Part model, mm, in its own coordinate system. A direction names the side the tool comes from. Give positions to 0.01 mm unless a question says otherwise; leave off trailing zeros. Order: outer loops, then holes, each group sorted by start corner. A loop starts at its lowest first (then second) coordinate and runs counter-clockwise, first axis right, second up. Notation, with made-up numbers: (66.5, 58) - (104.5, 58) arc R26 ccw to (104.5, 84) - close; hole circle Ø2 at (78, 85.5). An arc over 180 degrees is marked (long way). One line per item, written item: value.
```python
from build123d import *

# Parameters (mm, degrees)
BOSS_EXTRUDE1_DEPTH = 3


with BuildPart() as part:
    # Sketch1 → Boss-Extrude1 (new body)
    with BuildSketch(Plane.XY):
        Polygon((-112.34268018, 49.584121622), (-112.34268018, 23.584121622), (-115.34268018, 23.584121622), (-115.34268018, -26.415878378), (-112.34268018, -26.415878378), (-112.34268018, -52.415878378), (112.65731982, -52.415878378), (112.65731982, -26.415878378), (115.65731982, -26.415878378), (115.65731982, 23.584121622), (112.65731982, 23.584121622), (112.65731982, 49.584121622), align=None)
        with BuildLine():
            Line((13.274286272, -45.008836488), (13.301852176, -45.03203797))
            add(Edge.make_bspline(
                [(13.301852176, -45.03203797), (13.302434824, -45.031895887), (13.303594926, -45.031612989), (13.310345597, -45.026788399), (13.327424294, -45.013559601), (13.368373413, -44.979806794), (13.432345907, -44.924692433), (13.489247142, -44.874546261), (13.518732521, -44.84808225), (13.533463875, -44.834860418)],
                knots=[0, 0, 0, 0, 0.083775212, 0.166803477, 0.250583378, 0.499711324, 0.748903893, 0.874548479, 1, 1, 1, 1], degree=3))
            ThreePointArc((13.533463875, -44.834860418), (14.561847159, -43.83964014), (15.516962395, -42.773905432))
            ThreePointArc((15.516962395, -42.773905432), (30.145326147, -17.328936846), (35.253292189, 11.573383741))
            ThreePointArc((35.253292189, 11.573383741), (34.303607008, 26.14987852), (31.427393187, 40.471313366))
            ThreePointArc((31.427393187, 40.471313366), (30.556136604, 41.977838946), (29.052246095, 42.853636122))
            ThreePointArc((29.052246095, 42.853636122), (0.16598909, 46.766690687), (-28.731940535, 42.940791684))
            ThreePointArc((-28.731940535, 42.940791684), (-30.238466115, 42.069535101), (-31.114263292, 40.565644593))
            ThreePointArc((-31.114263292, 40.565644593), (-34.033665807, 26.252951242), (-35.027317855, 11.679387588))
            ThreePointArc((-35.027317855, 11.679387588), (-30.00656127, -17.238210094), (-15.455020905, -42.727190564))
            ThreePointArc((-15.455020905, -42.727190564), (-14.50312489, -43.795801606), (-13.477748449, -44.794119559))
            add(Edge.make_bspline(
                [(-13.477748449, -44.794119559), (-13.467950877, -44.802979196), (-13.448447729, -44.820615282), (-13.419486181, -44.846490582), (-13.372927905, -44.887713721), (-13.313203528, -44.93946889), (-13.269741808, -44.975508675), (-13.250245048, -44.990563249), (-13.247902102, -44.991518213), (-13.246732606, -44.991994889)],
                knots=[0, 0, 0, 0, 0.083817862, 0.166848714, 0.250507589, 0.499664298, 0.748829297, 0.874626478, 1, 1, 1, 1], degree=3))
            Line((-13.246732606, -44.991994889), (-13.219096838, -44.968876668))
            ThreePointArc((-13.219096838, -44.968876668), (0.020078677, -49.971995234), (13.274286272, -45.008836488))
        make_face(mode=Mode.SUBTRACT)
    extrude(amount=BOSS_EXTRUDE1_DEPTH)


solid = part.part
```
1) Cut at B-B, the plane x = -3.5. Give the cut face in (y, z).
Outcome:
outline: (-52.42, 0) - (-49.66, 0) - (-49.66, 3) - (-52.42, 3) - close; (46.71, 0) - (49.58, 0) - (49.58, 3) - (46.71, 3) - close
2) Pin check, flat tips, straight feed: pin 1 (8 mm diameter, centred on x = -3, y = -42, fed in from -Z); pin 2 (1.5 mm diameter, centred on x = 114, z = 1.5, fed in from -Y); pin 3 (1.5 mm diameter, centred on y = 33.5, z = 1, fed in from -X). Stop position of each tip, or through.
Outcome:
pin 1: passes through
pin 2: stops at y = -26.42
pin 3: stops at x = -112.34
3) Drill centre lines: line 1 along X through (y, z) = (10, 1.5); line 2 along X through (y, z) = (-24.5, 1.75); line 3 along Y through (x, z) = (-19, 1.2). Where is each one in solid material? Low to high. Write a range as from..to.
Outcome:
line 1: x = -115.34..-35.01, 35.24..115.66
line 2: x = -115.34..-27.01, 27.16..115.66
line 3: y = -52.42..-38.14, 45.11..49.58
4) Which spindle directions (+Z, -Z, +X, -X, +Y, -Y) get a long thin tool onto all of the face, cutting with end or side? Do faces 4 (the cylindrical face through (-0.18, -49.97, 1.48)), 5 (the flat face through (-27, -35, 3)). Say none if no direction does.
Outcome:
face 4: +Z, -Z
face 5: +Z, +X, -X, +Y, -Y
5) Mould opens along X. For faces 1 (the cylindrical face through (-34, 26.5, 1.5)), 2 (the flat face through (-27, -35, 0)), 3 (the cylindrical face through (-30.145, -16.849, 1.479)) say: released by +X, released by -X, zero draft, split by the parting line, or undercut.
Outcome:
face 1: undercut
face 2: zero draft
face 3: undercut
6) Cut at A-A, the plane y = 27. Give the cut face in (x, z).
Outcome:
outline: (-112.34, 0) - (-33.93, 0) - (-33.93, 3) - (-112.34, 3) - close; (34.19, 0) - (112.66, 0) - (112.66, 3) - (34.19, 3) - close
